Could you check a few things on this drawing? It's one solid part, dimensions in mm from its lowest x, y, z. Round coordinates to 2 decimals unless told otherwise and drop trailing zeros. Write each loop counter-clockwise with the first axis right and the second up, starting at its lowest first coordinate (ties: lowest second). Pieces come first, ordered by that corner, then holes. Notation, with made-up numbers: (12.25, 48.5) -> (45.25, 48.5) arc R29 cw to (45.25, 82.5) -> close; hole circle Ø9 at (11.25, -31.5). An arc over 180 degrees is marked (long way). Answer in a Markdown table with one row per item.
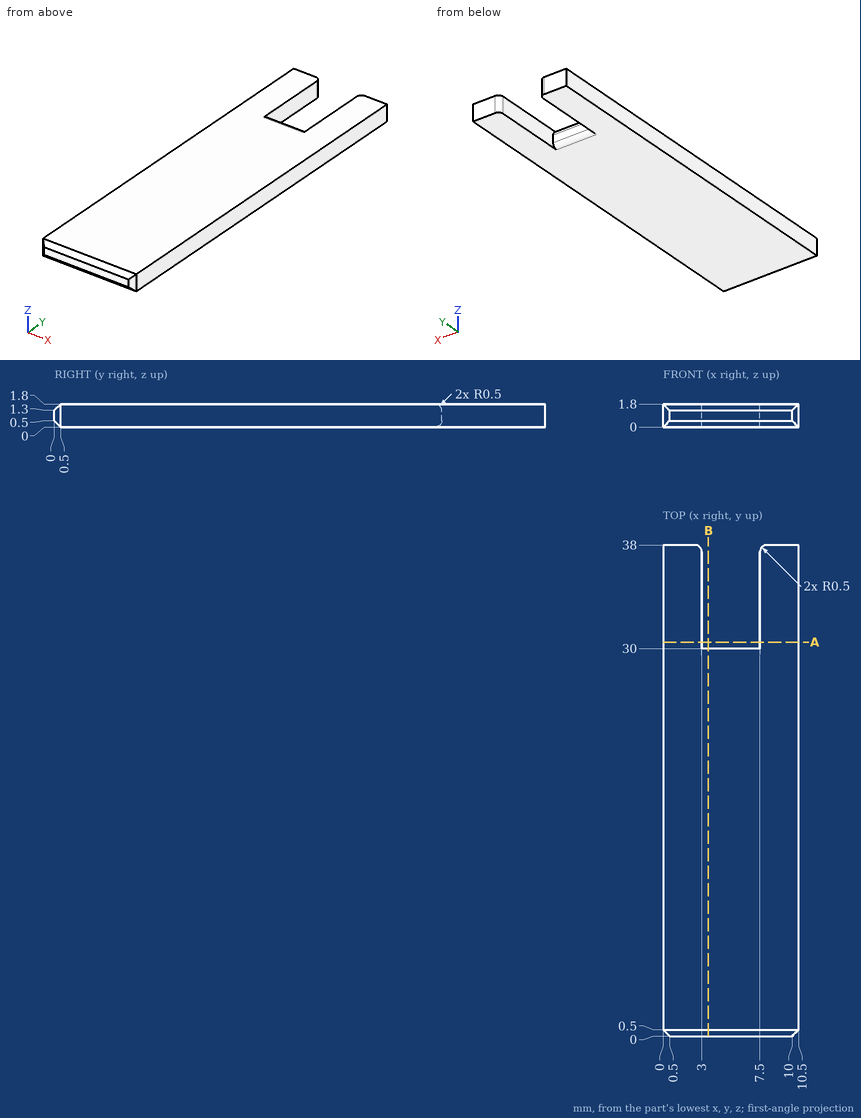
1) I want a section at A-A, the plane y = 30.5. List the corners of the cut face in (x, z) for me.
Response:
| item | result |
|---|---|
| outline | (0, 0) -> (3, 0) -> (3, 1.8) -> (0, 1.8) -> close; (7.5, 0) -> (10.5, 0) -> (10.5, 1.8) -> (7.5, 1.8) -> close |
2) I need wall thicknesses on line 1 (X direction, y = 31, z = 1.5); line 2 (Y direction, x = 7, z = 0.55); line 3 (Y direction, x = 5, z = 0.35). Which ranges of each line are inside material? Lowest first, please. Write a range as [from, to].
Response:
| item | result |
|---|---|
| line 1 | x = [0, 3], [7.5, 10.5] |
| line 2 | y = [0, 30] |
| line 3 | y = [0.15, 29.98] |
3) I want a section at B-B, the plane x = 3.5. List the corners of the cut face in (y, z) for me.
Response:
| item | result |
|---|---|
| outline | (0, 0.5) -> (0.5, 0) -> (29.5, 0) arc R0.5 ccw to (30, 0.5) -> (30, 1.3) arc R0.5 ccw to (29.5, 1.8) -> (0.5, 1.8) -> (0, 1.3) -> close |
